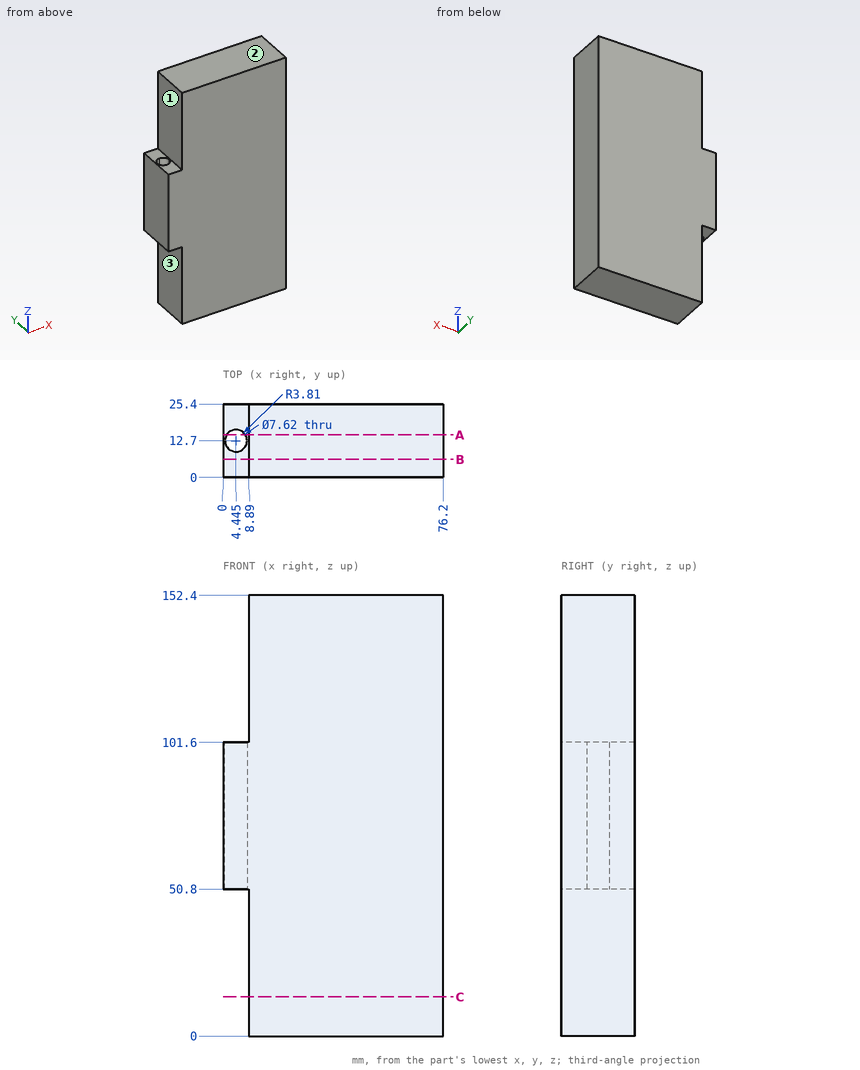
Could you check a few things on this drawing? It's one solid part, dimensions in mm from its lowest x, y, z. A direction names the side the tool comes from. Round coordinates to 2 decimals unless told otherwise and drop trailing zeros. Order: outer loops, then holes, each group sorted by start corner. A loop starts at its lowest first (then second) coordinate and runs counter-clockwise, first axis right, second up.
Q1. Please list where these lines run through material, in increasing order: probe 1 along X at (y, z) = (12.7, 66) (3 decimals); probe 2 along X at (y, z) = (16, 94.5); probe 3 along X at (y, z) = (8, 40).
Geometry says:
probe 1: x = 0 to 0.635, 8.255 to 76.2
probe 2: x = 0 to 2.54, 6.35 to 76.2
probe 3: x = 8.89 to 76.2
Q2. Imagine slicing it at A-A, the plane y = 14.75. List the corners of the cut face in (x, z) for me, then the cut area to 3 significant figures.
Geometry says:
outline: (0, 50.8) - (1.23, 50.8) - (1.23, 101.6) - (0, 101.6) - close; (7.66, 50.8) - (8.89, 50.8) - (8.89, 0) - (76.2, 0) - (76.2, 152.4) - (8.89, 152.4) - (8.89, 101.6) - (7.66, 101.6) - close
area: 10,400 mm2
Q3. Which directions (+Z, -Z, +X, -X, +Y, -Y) give clear straight access to the entire face, cutting with the end or side of a thin tool? Please do the marked faces 1, 2 and 3.
Geometry says:
face 1: +Z, -X, +Y, -Y
face 2: +Z, +X, -X, +Y, -Y
face 3: -Z, -X, +Y, -Y
Q4. Imagine slicing it at C-C, the plane z = 13.5. List the corners of the cut face in (x, y) for me.
Geometry says:
outline: (8.89, 0) - (76.2, 0) - (76.2, 25.4) - (8.89, 25.4) - close
Q5. I'm going to push flat-ended pins straight in: P1, Ø6, axis at y = 21, z = 121, coming from the -X side; P2, Ø2.5, axis at x = 3.5, y = 6.5, coming from the -Z side. Where does each tip first touch, or does it pass through?
Geometry says:
P1: stops at x = 8.89
P2: stops at z = 50.8
Q6. Imagine slicing it at B-B, the plane y = 6.25. List the corners of the cut face in (x, z) for me, then the cut area to 3 significant figures.
Geometry says:
outline: (0, 50.8) - (8.89, 50.8) - (8.89, 0) - (76.2, 0) - (76.2, 152.4) - (8.89, 152.4) - (8.89, 101.6) - (0, 101.6) - close
area: 10,700 mm2
